Geometry check sheet. Reference: the model listing, model coordinates, mm. Face numbers are marked on the shaded views. Round coordinates to 2 decimals unless told otherwise and drop trailing zeros. Order: outer loops, then holes, each group sorted by start corner. A loop starts at its lowest first (then second) coordinate and runs counter-clockwise, first axis right, second up. Notation, with made-up numbers: (76, 30.25) -> (98, 30.25) arc R21 ccw to (98, 61.25) -> close; hole circle Ø3 at (43, 32.5). An arc over 180 degrees is marked (long way). Use a Markdown table: item, result. Add a question column.
Item 1: Sectioned sample at A-A, the plane x = 36. Record the cut outline in (y, z) (3 decimals), and give its area (3 significant figures).
Item 2: Mould release check, pull along Y, two halves, no side actions. Record for the marked faces 1 and 2: pulls with the +Y half, pulls with the -Y half, needs draft (parallel to the pull), parting line crosses it, or undercut.
Item 3: Sectioned sample at B-B, the plane z = 5. Record the cut outline in (x, y) (3 decimals).
Item 4: Material ranges on probe 1 along X at (y, z) = (14, 5.75) (3 decimals); probe 2 along Z at (x, y) = (-33, -26), recorded low to high. Write a range as [from, to].
Item 5: Gauge pin test, flat end, axial feed: pin 1 Ø1 at (x, y) = (-14, 15.5) entering from +Z. Record the tip position at first contact, or that the pin passes through.
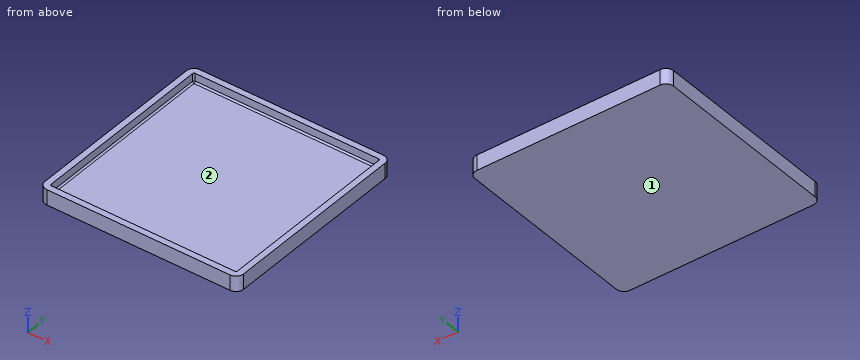
Solid Edge part; units mm, degrees
sketch "Sketch1" plane through (0, 0, 0) normal (0, 0, 1) x (1, 0, 0)
  line L0 (-38.735, -38.735) -> (38.735, -38.735)
  line L1 (38.735, -38.735) -> (38.735, 38.735)
  line L2 (38.735, 38.735) -> (-38.735, 38.735)
  line L3 (-38.735, 38.735) -> (-38.735, -38.735)
extrude "Protrusion1" add sketch "Sketch1" along normal blind 2.54
sketch "Sketch2" plane through (0, 0, 0) normal (0, 0, 1) x (1, 0, 0)
  line L0 (-41.275, -41.275) -> (41.275, -41.275)
  line L1 (41.275, -41.275) -> (41.275, 41.275)
  line L2 (41.275, 41.275) -> (-41.275, 41.275)
  line L3 (-41.275, 41.275) -> (-41.275, -41.275)
  line L4 (-38.735, -38.735) -> (38.735, -38.735)
  line L5 (38.735, -38.735) -> (38.735, 38.735)
  line L6 (38.735, 38.735) -> (-38.735, 38.735)
  line L7 (-38.735, 38.735) -> (-38.735, -38.735)
extrude "ExtrudedProtrusion_2" add sketch "Sketch2" along normal blind 6.35
fillet "Round_1" radius 3.175 4 edges at (41.275, -41.275, 3.175) (41.275, 41.275, 3.175) (-41.275, 41.275, 3.175) (-41.275, -41.275, 3.175)
fillet "Round_2" radius 0.635 4 edges at (-38.735, 0, 2.54) (0, -38.735, 2.54) (38.735, 0, 2.54) (0, 38.735, 2.54)
fillet "Round_3" radius 0.635 8 edges at (-38.735, 38.735, 4.7625) (-38.549, 38.549, 2.726) (-38.549, -38.549, 2.726) (-38.735, -38.735, 4.7625) (38.735, -38.735, 4.7625) (38.549, -38.549, 2.726) (38.735, 38.735, 4.7625) (38.549, 38.549, 2.726)
Found:
| question | item | result |
|---|---|---|
| 1 | outline | (-41.275, 0) -> (41.275, 0) -> (41.275, 6.35) -> (38.735, 6.35) -> (38.735, 3.175) arc R0.635 cw to (38.1, 2.54) -> (-38.1, 2.54) arc R0.635 cw to (-38.735, 3.175) -> (-38.735, 6.35) -> (-41.275, 6.35) -> close |
| 1 | area | 229 mm2 |
| 2 | face 1 | needs draft |
| 2 | face 2 | undercut |
| 3 | outline | (-41.275, -38.1) arc R3.175 ccw to (-38.1, -41.275) -> (38.1, -41.275) arc R3.175 ccw to (41.275, -38.1) -> (41.275, 38.1) arc R3.175 ccw to (38.1, 41.275) -> (-38.1, 41.275) arc R3.175 ccw to (-41.275, 38.1) -> close; hole (-38.735, -38.1) arc R0.635 ccw to (-38.1, -38.735) -> (38.1, -38.735) arc R0.635 ccw to (38.735, -38.1) -> (38.735, 38.1) arc R0.635 ccw to (38.1, 38.735) -> (-38.1, 38.735) arc R0.635 ccw to (-38.735, 38.1) -> close |
| 4 | probe 1 | x = [-41.275, -38.735], [38.735, 41.275] |
| 4 | probe 2 | z = [0, 2.54] |
| 5 | pin 1 | stops at z = 2.54 |
